CAD build for the part. Positions are in the model's coordinates, mm. Face numbers are marked on the shaded views. A direction names the side the tool comes from. Round coordinates to 2 decimals unless told otherwise and drop trailing zeros. Order: outer loops, then holes, each group sorted by start corner. A loop starts at its lowest first (then second) coordinate and runs counter-clockwise, first axis right, second up. Notation, with made-up numbers: (4.5, 63) -> (38.5, 63) arc R36 ccw to (38.5, 101) -> close; hole circle Ø6 at (22.25, -26). An arc over 180 degrees is marked (long way). Return JSON: item names as keys, results as strings. Group by question number.
Q1. Cut at B-B (z = 0). Write the cut outline in (x, y).
Q2. Which spindle directions (+Z, -Z, +X, -X, +Y, -Y) get a long thin tool onto all of the face, cutting with end or side? Do the marked faces 5, 6, 7 and 8. Say none if no direction does.
Q3. Probe line 1 along X through (y, z) = (5.55, 0); line 2 along Z through (x, y) = (0, 0.8); line 3 along Y through (x, z) = (-0.75, -0.8). List the from-to ranges inside material, lowest first.
Q4. Flat gauge pins, fed straight in: pin 1 (1.1 mm diameter, centred on x = 0, z = 0, fed in from +Y); pin 2 (0.6 mm diameter, centred on y = 1, z = -1, fed in from +X); pin 3 (2 mm diameter, centred on y = 6.5, z = -2, fed in from +X); pin 4 (1.6 mm diameter, centred on y = 3.5, z = 0.5, fed in from -X). Where does each tip first touch, or does it go through?
Q5. Cut at D-D (x = 0). Write the cut outline in (y, z).
Q6. Mould opens along Y. For the marked faces 1, 2, 3 and 4 say: +Y half, -Y half, draft (parallel to the pull), parting line (faces both ways), or undercut.
Q7. Cut at A-A (x = 2). Write the cut outline in (y, z).
Q8. Cut at C-C (y = 3.25). Write the cut outline in (x, z).
from build123d import *

# Parameters (mm, degrees)
SKETCH1_R           = 0.9
BOSS_EXTRUDE1_DEPTH = 7
CUT_EXTRUDE1_REACH  = 16.739
SKETCH2_W           = 6
SKETCH2_H           = 3.2
SKETCH3_W           = 2.5
SKETCH3_H           = 2
CUT_EXTRUDE2_DEPTH  = 4
CHAMFER1_SIZE       = 1


with BuildPart() as part:
    # Sketch1 → Boss-Extrude1 (new body)
    with BuildSketch(Plane(origin=(0, 0, 0), x_dir=(1, 0, 0), z_dir=(0, 1, 0))):
        with BuildLine():
            Line((-1, 2), (7, 2))
            Line((7, 2), (7, 4))
            Line((7, 4), (11.5, 4))
            Line((11.5, 4), (11.5, 2))
            Line((11.5, 2), (11.5, -2))
            Line((11.5, -2), (-1, -2))
            ThreePointArc((-1, -2), (-3, 0), (-1, 2))
        make_face()
        with Locations(Location((0, 0, 0), (0, 0, 270))):
            Circle(SKETCH1_R, mode=Mode.SUBTRACT)
    extrude(amount=BOSS_EXTRUDE1_DEPTH)

    # Sketch2 → Cut-Extrude1 (cut, up to next)
    with BuildSketch(Plane.XY.offset(2), mode=Mode.PRIVATE) as cut_extrude1_sk1:
        with Locations((0, 3.5)):
            Rectangle(SKETCH2_W, SKETCH2_H)
    cut_extrude1_tool1 = extrude(cut_extrude1_sk1.sketch, amount=-CUT_EXTRUDE1_REACH, mode=Mode.PRIVATE) & part.part
    add(cut_extrude1_tool1.solids().sort_by_distance((0, 3.5, 2))[0], mode=Mode.SUBTRACT)

    # Sketch3 → Cut-Extrude2 (cut)
    with BuildSketch(Plane(origin=(11.5, 0, 0), x_dir=(0, 0, -1), z_dir=(1, 0, 0))):
        with Locations((2.4, 6)):
            Rectangle(SKETCH3_W, SKETCH3_H)
        with Locations((0.9, 1)):
            Rectangle(SKETCH3_W, SKETCH3_H)
    extrude(amount=-CUT_EXTRUDE2_DEPTH, mode=Mode.SUBTRACT)

    # Chamfer1
    chamfer1_edges = [part.edges().sort_by_distance(p)[0] for p in [
        (11.5, 3.5, 2),
    ]]
    chamfer(chamfer1_edges, length=CHAMFER1_SIZE)


solid = part.part
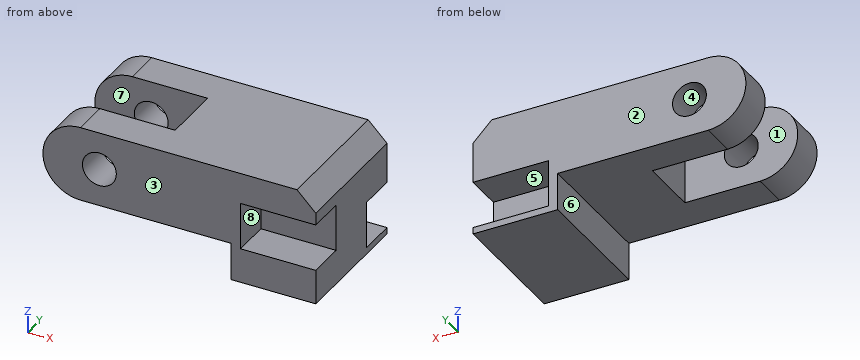
Solution:
{
 "1": {"outline": "(-3, 0) -> (-0.9, 0) -> (-0.9, 1.9) -> (-3, 1.9) -> close; (-3, 5.1) -> (-0.9, 5.1) -> (-0.9, 7) -> (-3, 7) -> close; (0.9, 0) -> (7.5, 0) -> (7.5, 2) -> (11.5, 2) -> (11.5, 7) -> (0.9, 7) -> (0.9, 5.1) -> (3, 5.1) -> (3, 1.9) -> (0.9, 1.9) -> close"},
 "2": {"face 5": "+X, +Y", "face 6": "-Z, -X, +Y, -Y", "face 7": "+Z, -Z, -X", "face 8": "+X, -Y"},
 "3": {"line 1": "x = -3 to -0.9, 0.9 to 11.5", "line 2": "z = -2 to -0.9, 0.9 to 2", "line 3": "y = 0 to 1.9, 5.1 to 7"},
 "4": {"pin 1": "passes through", "pin 2": "stops at x = 7.5", "pin 3": "stops at x = 11.5", "pin 4": "stops at x = 3"},
 "5": {"outline": "(0, -2) -> (1.9, -2) -> (1.9, -0.9) -> (0, -0.9) -> close; (0, 0.9) -> (1.9, 0.9) -> (1.9, 2) -> (0, 2) -> close; (5.1, -2) -> (7, -2) -> (7, -0.9) -> (5.1, -0.9) -> close; (5.1, 0.9) -> (7, 0.9) -> (7, 2) -> (5.1, 2) -> close"},
 "6": {"face 1": "undercut", "face 2": "+Y half", "face 3": "-Y half", "face 4": "draft"},
 "7": {"outline": "(0, -2) -> (1.9, -2) -> (1.9, 2) -> (0, 2) -> close; (5.1, -2) -> (7, -2) -> (7, 2) -> (5.1, 2) -> close"},
 "8": {"outline": "(3, -2) -> (7, -2) -> (7, -4) -> (11.5, -4) -> (11.5, 1) -> (10.5, 2) -> (3, 2) -> close"}
}
